Source: CAD feature listing. Evaluate the final solid. Frame: model axes, mm. Round coordinates to 2 decimals unless told otherwise and drop trailing zeros. Loops run counter-clockwise (first coordinate to the right, second up) from the corner with the lowest first, then second, coordinate; pieces in that order, holes last. Notation, with made-up numbers: M -9,37 L 11,37 A16 ccw 11,58 Z; hole C 88.5,12 d1. An arc over 180 degrees is marked long. Answer as CSV lines item,"result". Start each with the question number.
Autodesk Inventor part; units mm, degrees
ref_plane "YZ Plane" through (0, 0, 0) normal (1, 0, 0) x (0, 1, 0)
ref_plane "XZ Plane" through (0, 0, 0) normal (0, 1, 0) x (-1, 0, 0)
ref_plane "XY Plane" through (0, 0, 0) normal (0, 0, 1) x (1, 0, 0)
sketch "Sketch3" plane through (0, 0, 0) normal (1, 0, 0) x (0, 1, 0)
  line L0 (0, 57) -> (0, 13)
  circle A0 centre (84, 35) radius 4.25
  line L1 (84, 35) -> (56.36, 35)
  line L2 (96, 53.4391) -> (92.6159, 55.2427)
  arc A1 (94.3473, 15.5852) -> (92.6159, 55.2427) centre (84, 35) ccw
  line L3 (84, 35) -> (71.3, 35)
  arc A2 (84, 13) -> (84, 57) centre (84, 35) ccw
  line L4 (84, 35) -> (84, 57)
  line L5 (0, 57) -> (84, 57)
  line L6 (84, 13) -> (0, 13)
  point P0 (0, 0)
  point P1 (84, 10.0705)
  point P2 (74.9172, 64.6754)
  dimension "d31" = 8.5
  dimension "d33" = 27.64
  dimension "d35" = 12.7
  dimension "d41" = 84
extrude "Extrusion3" add sketch "Sketch3" along normal blind 6
properties part number "Suporte Motor"
1) Contact query for a flat-ended pin moving along its axis: pin 1 Ø1.5 at (y, z) = (89, 23.5) entering from -X. Output: stop coordinate, or through.
2) Ray query, line 1 along Y through (x, z) = (2.75, 35); line 2 along Z through (x, y) = (0.95, 81.5); line 3 along Y through (x, z) = (2.6, 37.5). Return the intervals inside material, ascending.
3) Section B-B, the plane z = 35. Return loops of the section in (x, y).
4) Section A-A, the plane x = 1.2. Return loops of the section in (y, z), and give its area (3 significant figures).
5) Mould query, pull axis Z, two halves, no side actions, for faces 1 (the flat face through (3, 43, 13)), 2 (the cylindrical face through (2.958, 83.447, 30.786)), 3 (the flat face through (6, 52, 35)). Classes: pulls with the +Z half, pulls with the -Z half, needs draft (parallel to the pull), parting line crosses it, or undercut.
6) Section C-C, the plane y = 91. Return loops of the section in (x, z).
Findings below:
1,pin 1,"x = 0"
2,line 1,"0 to 79.75, 88.25 to 106"
2,line 2,"13 to 31.56, 38.44 to 57"
2,line 3,"0 to 80.56, 87.44 to 105.86"
3,outline,"M 0,0 L 6,0 L 6,79.75 L 0,79.75 Z; M 0,88.25 L 6,88.25 L 6,106 L 0,106 Z"
4,outline,"M 0,13 L 84,13 A22 ccw 94.35,15.59 A22 ccw 92.62,55.24 A22 ccw 84,57 L 0,57 Z; hole C 84,35 d8.5"
4,area,"4,400 mm²"
5,face 1,"pulls with the -Z half"
5,face 2,"undercut"
5,face 3,"needs draft"
6,outline,"M 0,14.14 L 6,14.14 L 6,55.86 L 0,55.86 Z"
